The listing builds one solid part. Answer for the finished solid, in the listing's coordinates (mm). Face numbers are marked on the shaded views. A direction names the side the tool comes from. Round coordinates to 2 decimals unless told otherwise and drop trailing zeros. Loops run counter-clockwise (first coordinate to the right, second up) from the corner with the lowest first, then second, coordinate; pieces in that order, holes last. Notation, with made-up numbers: (2, 73.25) - (39, 73.25) arc R30 ccw to (39, 108.25) - close; hole circle Ø8 at (20, 0). An arc over 180 degrees is marked (long way). Write item = value, one per line. Start each with the question number.
1) Given pin 1 Ø1.5 at (x, z) = (-6, 2) entering from +Y; pin 2 Ø10 at (x, y) = (-4.5, 12.5) entering from -Z, each flat-ended and moving along its own axis, determine where each tip first touches the part or whether it passes through.
2) For a pull along Y with two mould halves and no side action, classify the marked faces 4, 5 and 6 as released by +Y, released by -Y, zero draft, split by the parting line, or undercut.
3) Section B-B, the plane x = -7 is taken. Determine the outline of the cut face in (y, z).
4) A tool of negligible diameter and unlimited length cuts with its end or side. For the marked faces 1, 2 and 3, from which of +Z, -Z, +X, -X, +Y, -Y can it reach the whole face along a straight path? Write none if from no direction.
5) Section D-D, the plane z = 3 is taken. Determine the outline of the cut face in (x, y), and give its area (3 significant figures).
6) Section A-A, the plane y = 9.25 is taken. Determine the outline of the cut face in (x, z), and give its area (3 significant figures).
7) Section C-C, the plane y = 7 is taken. Determine the outline of the cut face in (x, z), and give its area (3 significant figures).
8) Straight lines are drawn through the part: line 1 along Y through (x, z) = (-12.75, -8.5); line 2 along X through (y, z) = (8, -6.25); line 3 along X through (y, z) = (12, -0.5). For each, find the intervals that lie inside material, in ascending order.
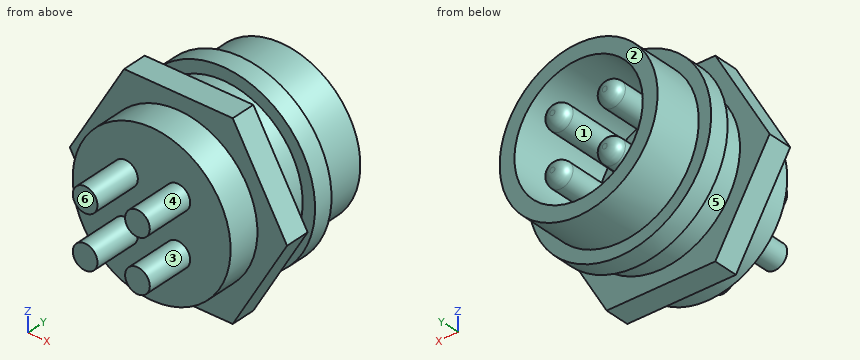
from build123d import *

# Parameters (mm, degrees)
SZKIC1_R                                = 8
DODANIE_WYCI_GNI_CIE1_DEPTH             = 15.75
SZKIC2_R                                = 6.5
WYTNIJ_WYCI_GNI_CIE1_DEPTH              = 10
DODANIE_WYCI_GNI_CIE2_START             = -2
SZKIC4_R                                = 9.25
SZKIC4_R_2                              = 8
DODANIE_WYCI_GNI_CIE2_DEPTH             = 2
SZKIC5_R                                = 1.25
DODANIE_WYCI_GNI_CIE3_DEPTH             = 4.9
DODANIE_WYCI_GNI_CIE3_DIRECTION_2_REACH = 27.08
ZAOKR_GLENIE1_R                         = 1
DODANIE_WYCI_GNI_CIE4_START             = 2.5
SZKIC6_R                                = 8
DODANIE_WYCI_GNI_CIE4_DEPTH             = 2.5


with BuildPart() as part:
    # Szkic1 → Dodanie-wyciągnięcie1 (new body)
    with BuildSketch(Plane(origin=(0, 0, 0), x_dir=(1, 0, 0), z_dir=(0, 1, 0))):
        with Locations(Location((-6.199930539, 2.677242733, 0), (0, 0, 270))):
            Circle(SZKIC1_R)
    extrude(amount=DODANIE_WYCI_GNI_CIE1_DEPTH)

    # Szkic2 → Wytnij-wyciągnięcie1 (cut)
    with BuildSketch(Plane(origin=(0, 15.75, 0), x_dir=(1, 0, 0), z_dir=(0, 1, 0))):
        with Locations(Location((-6.199930539, 2.677242733, 0), (0, 0, 270))):
            Circle(SZKIC2_R)
    extrude(amount=-WYTNIJ_WYCI_GNI_CIE1_DEPTH, mode=Mode.SUBTRACT)

    # Szkic4 → Dodanie-wyciągnięcie2 (add)
    with BuildSketch(Plane(origin=(0, 10.75, 0), x_dir=(1, 0, 0), z_dir=(0, 1, 0)).offset(DODANIE_WYCI_GNI_CIE2_START)):
        with Locations(Location((-6.199930539, 2.677242733, 0), (0, 0, 270))):
            Circle(SZKIC4_R)
        with Locations(Location((-6.199930539, 2.677242733, 0), (0, 0, 270))):
            Circle(SZKIC4_R_2, mode=Mode.SUBTRACT)
    extrude(amount=DODANIE_WYCI_GNI_CIE2_DEPTH)

    # Szkic5 → Dodanie-wyciągnięcie3 (add)
    with BuildSketch(Plane.XZ):
        with Locations(Location((-8.849930539, -0.027242733, 0), (0, 0, 270))):
            Circle(SZKIC5_R)
        with Locations(Location((-3.549930539, -0.027242733, 0), (0, 0, 270))):
            Circle(SZKIC5_R)
        with Locations(Location((-3.549930539, -5.327242733, 0), (0, 0, 270))):
            Circle(SZKIC5_R)
        with Locations(Location((-8.849930539, -5.327242733, 0), (0, 0, 270))):
            Circle(SZKIC5_R)
    extrude(amount=DODANIE_WYCI_GNI_CIE3_DEPTH)

    # Dodanie-wyciągnięcie3 direction 2: up to this face of the body (flat: up to its plane)
    dodanie_wyci_gni_cie3_direction_2_end = Plane(part.part.faces().sort_by_distance((-6.199930539, 15.75, -10.450968563))[0])
    # Szkic5 → Dodanie-wyciągnięcie3 direction 2 (add, up to the picked face)
    with BuildSketch(Plane.XZ, mode=Mode.PRIVATE) as dodanie_wyci_gni_cie3_direction_2_sk1:
        with Locations(Location((-8.849930539, -0.027242733, 0), (0, 0, 270))):
            Circle(SZKIC5_R)
    dodanie_wyci_gni_cie3_direction_2_tool1 = split(extrude(dodanie_wyci_gni_cie3_direction_2_sk1.sketch, amount=-DODANIE_WYCI_GNI_CIE3_DIRECTION_2_REACH, mode=Mode.PRIVATE), bisect_by=dodanie_wyci_gni_cie3_direction_2_end, keep=Keep.BOTH, mode=Mode.PRIVATE)
    # Szkic5 → Dodanie-wyciągnięcie3 direction 2 (add, up to the picked face)
    with BuildSketch(Plane.XZ, mode=Mode.PRIVATE) as dodanie_wyci_gni_cie3_direction_2_sk2:
        with Locations(Location((-3.549930539, -0.027242733, 0), (0, 0, 270))):
            Circle(SZKIC5_R)
    dodanie_wyci_gni_cie3_direction_2_tool2 = split(extrude(dodanie_wyci_gni_cie3_direction_2_sk2.sketch, amount=-DODANIE_WYCI_GNI_CIE3_DIRECTION_2_REACH, mode=Mode.PRIVATE), bisect_by=dodanie_wyci_gni_cie3_direction_2_end, keep=Keep.BOTH, mode=Mode.PRIVATE)
    # Szkic5 → Dodanie-wyciągnięcie3 direction 2 (add, up to the picked face)
    with BuildSketch(Plane.XZ, mode=Mode.PRIVATE) as dodanie_wyci_gni_cie3_direction_2_sk3:
        with Locations(Location((-3.549930539, -5.327242733, 0), (0, 0, 270))):
            Circle(SZKIC5_R)
    dodanie_wyci_gni_cie3_direction_2_tool3 = split(extrude(dodanie_wyci_gni_cie3_direction_2_sk3.sketch, amount=-DODANIE_WYCI_GNI_CIE3_DIRECTION_2_REACH, mode=Mode.PRIVATE), bisect_by=dodanie_wyci_gni_cie3_direction_2_end, keep=Keep.BOTH, mode=Mode.PRIVATE)
    # Szkic5 → Dodanie-wyciągnięcie3 direction 2 (add, up to the picked face)
    with BuildSketch(Plane.XZ, mode=Mode.PRIVATE) as dodanie_wyci_gni_cie3_direction_2_sk4:
        with Locations(Location((-8.849930539, -5.327242733, 0), (0, 0, 270))):
            Circle(SZKIC5_R)
    dodanie_wyci_gni_cie3_direction_2_tool4 = split(extrude(dodanie_wyci_gni_cie3_direction_2_sk4.sketch, amount=-DODANIE_WYCI_GNI_CIE3_DIRECTION_2_REACH, mode=Mode.PRIVATE), bisect_by=dodanie_wyci_gni_cie3_direction_2_end, keep=Keep.BOTH, mode=Mode.PRIVATE)
    add(dodanie_wyci_gni_cie3_direction_2_tool1.solids().sort_by(Axis((-8.849931, 0, -0.027243), (0, 1, 0)))[0])
    add(dodanie_wyci_gni_cie3_direction_2_tool2.solids().sort_by(Axis((-3.549931, 0, -0.027243), (0, 1, 0)))[0])
    add(dodanie_wyci_gni_cie3_direction_2_tool3.solids().sort_by(Axis((-3.549931, 0, -5.327243), (0, 1, 0)))[0])
    add(dodanie_wyci_gni_cie3_direction_2_tool4.solids().sort_by(Axis((-8.849931, 0, -5.327243), (0, 1, 0)))[0])

    # Zaokrąglenie1
    zaokr_glenie1_edges = [part.edges().sort_by_distance(p)[0] for p in [
        (-8.849930539, 15.75, 1.222757267),
        (-3.549930539, 15.75, 1.222757267),
        (-3.549930539, 15.75, -4.077242733),
        (-8.849930539, 15.75, -4.077242733),
    ]]
    fillet(zaokr_glenie1_edges, radius=ZAOKR_GLENIE1_R)

    # Szkic6 → Dodanie-wyciągnięcie4 (add)
    with BuildSketch(Plane(origin=(0, 5.75, 0), x_dir=(-1, 0, 0), z_dir=(0, -1, 0)).offset(DODANIE_WYCI_GNI_CIE4_START)):
        Polygon((17.202288313, 2.677242733), (11.701109426, 12.205564067), (0.698751652, 12.205564067), (-4.802427235, 2.677242733), (0.698751652, -6.851078601), (11.701109426, -6.851078601), align=None)
        with Locations(Location((6.199930539, 2.677242733, 0), (0, 0, 90))):
            Circle(SZKIC6_R, mode=Mode.SUBTRACT)
    extrude(amount=-DODANIE_WYCI_GNI_CIE4_DEPTH)


solid = part.part
Geometry check:
q1.pin_1 = 5.75
q1.pin_2 = -11.93
q2.face_4 = zero draft
q2.face_5 = undercut
q2.face_6 = released by -Y
q3.outline = (0, -10.64) - (3.25, -10.64) - (3.25, -12.21) - (5.75, -12.21) - (5.75, -10.64) - (8.75, -10.64) - (8.75, -11.89) - (10.75, -11.89) - (10.75, -10.64) - (15.75, -10.64) - (15.75, -9.13) - (5.75, -9.13) - (5.75, 3.77) - (15.75, 3.77) - (15.75, 5.28) - (10.75, 5.28) - (10.75, 6.54) - (8.75, 6.54) - (8.75, 5.28) - (5.75, 5.28) - (5.75, 6.85) - (3.25, 6.85) - (3.25, 5.28) - (0, 5.28) - close
q4.face_1 = +Y
q4.face_2 = +Z, -Z, +X, -X, +Y
q4.face_3 = -Y
q5.outline = (-13.92, 3.25) - (-11.84, 3.25) - (-11.84, 0) - (-0.56, 0) - (-0.56, 3.25) - (1.52, 3.25) - (1.52, 5.75) - (-0.56, 5.75) - (-0.56, 8.75) - (1.1, 8.75) - (1.1, 10.75) - (-0.56, 10.75) - (-0.56, 15.75) - (-3.03, 15.75) - (-3.03, 5.75) - (-9.37, 5.75) - (-9.37, 15.75) - (-11.84, 15.75) - (-11.84, 10.75) - (-13.5, 10.75) - (-13.5, 8.75) - (-11.84, 8.75) - (-11.84, 5.75) - (-13.92, 5.75) - close
q5.area = 131 mm2
q6.outline = circle Ø18.5 at (-6.2, -2.68); circle Ø2.5 at (-8.85, -5.33); circle Ø2.5 at (-8.85, -0.03); circle Ø2.5 at (-3.55, -5.33); circle Ø2.5 at (-3.55, -0.03); hole circle Ø13 at (-6.2, -2.68)
q6.area = 156 mm2
q7.outline = circle Ø16 at (-6.2, -2.68); circle Ø2.5 at (-8.85, -5.33); circle Ø2.5 at (-8.85, -0.03); circle Ø2.5 at (-3.55, -5.33); circle Ø2.5 at (-3.55, -0.03); hole circle Ø13 at (-6.2, -2.68)
q7.area = 88.0 mm2
q8.line_1 = 3.25 to 5.75, 8.75 to 10.75
q8.line_2 = -13.36 to -11.63, -9.69 to -8.01, -4.39 to -2.71, -0.77 to 0.96
q8.line_3 = -13.9 to -12.32, -10.01 to -7.69, -4.71 to -2.39, -0.08 to 1.5
